Work out the finished part from the listing and answer in its coordinate system (mm). Face numbers are marked on the shaded views. A direction names the side the tool comes from. Coordinates: 2 decimals unless noted, no trailing zeros. Write each loop counter-clockwise with the first axis right and the second up, starting at its lowest first coordinate (ties: lowest second). Pieces come first, ordered by that corner, then holes. Notation, with made-up numbers: (58, -32.5) - (78, -32.5) arc R11 cw to (78, -18.5) - close; hole circle Ø2 at (37.25, 73). An arc over 180 degrees is marked (long way). Use a Markdown table: item, result. Add a question column.
(1) The part is cut by section A-A, the plane z = 6. Give the vertices of the cut face in (x, y) (3 decimals).
(2) Given pin 1 Ø6 at (x, y) = (-3, -27.5) entering from -Z; pin 2 Ø3 at (x, y) = (0, -1) entering from -Z; pin 3 Ø5.5 at (x, z) = (0.5, 9.5) entering from -Y (3 decimals), each flat-ended and moving along its own axis, determine where each tip first touches the part or whether it passes through.
(3) The part is cut by section C-C, the plane x = 0. Give the vertices of the cut face in (y, z) (3 decimals).
(4) Find the intervals of material crossed by line 1 (X direction, y = 0, z = -1); line 2 (X direction, y = -18, z = 12) (3 decimals); line 3 (Z direction, x = 3.75, y = -17) (3 decimals), in increasing order. Write a range as from..to.
(5) The part is cut by section D-D, the plane z = 20.65. Give the vertices of the cut face in (x, y) (3 decimals).
(6) For a pull along Z with two mould halves and no side action, classify the marked faces 4, 5 and 6 as released by +Z, released by -Z, zero draft, split by the parting line, or undercut.
(7) The part is cut by section B-B, the plane y = 0. Give the vertices of the cut face in (x, z) (3 decimals), then the cut area to 3 significant figures.
(8) A tool of negligible diameter and unlimited length cuts with its end or side. For the marked faces 1, 2 and 3, from which of +Z, -Z, +X, -X, +Y, -Y can it reach the whole face along a straight path? Write none if from no direction.
from build123d import *

# Parameters (mm, degrees)
BOSS_EXTRUDE1_DEPTH = 25.4
CUT_EXTRUDE1_DEPTH  = 9.5
SKETCH5_W           = 25.4
SKETCH5_H           = 42.164
BOSS_EXTRUDE2_DEPTH = 11.43
CUT_EXTRUDE2_REACH  = 53.538
CUT_EXTRUDE3_REACH  = 53.255
CUT_EXTRUDE4_DEPTH  = 20
SKETCH10_W          = 19.05
SKETCH10_H          = 19.05
CUT_EXTRUDE5_DEPTH  = 26.289
CUT_EXTRUDE6_REACH  = 55.322
SKETCH11_W          = 1.5875
SKETCH11_H          = 12.7
SKETCH12_R          = 0.9921875
CUT_EXTRUDE7_DEPTH  = 51.724378715
CUT_EXTRUDE8_REACH  = 52.836
SKETCH13_R          = 0.9921875


with BuildPart() as part:
    # Sketch2 → Boss-Extrude1 (new body)
    with BuildSketch(Plane.XY):
        Polygon((12.7, -6.35), (14.2875, -6.35), (14.2875, 6.35), (-14.2875, 6.35), (-14.2875, -6.35), (-12.7, -6.35), (-12.7, -35.814), (12.7, -35.814), align=None)
    extrude(amount=BOSS_EXTRUDE1_DEPTH)

    # Sketch3 → Cut-Extrude1 (cut)
    with BuildSketch(Plane.XY.offset(25.4)):
        with BuildLine():
            Line((2.003122562, 2.3), (2.003122562, -2.3))
            ThreePointArc((2.003122562, -2.3), (-3.05, 0), (2.003122562, 2.3))
        make_face()
    extrude(amount=-CUT_EXTRUDE1_DEPTH, mode=Mode.SUBTRACT)

    # Sketch5 → Boss-Extrude2 (add)
    with BuildSketch(Plane(origin=(0, 0, 0), x_dir=(-1, 0, 0), z_dir=(0, 0, -1))):
        with Locations((0, -14.732)):
            Rectangle(SKETCH5_W, SKETCH5_H)
    extrude(amount=BOSS_EXTRUDE2_DEPTH)

    # Sketch6 → Cut-Extrude2 (cut, up to next)
    with BuildSketch(Plane(origin=(12.7, 0, 0), x_dir=(0, 0, -1), z_dir=(1, 0, 0)), mode=Mode.PRIVATE) as cut_extrude2_sk1:
        Polygon((3.175, -35.814), (11.43, -23.01875), (11.43, -35.814), align=None)
    cut_extrude2_tool1 = extrude(cut_extrude2_sk1.sketch, amount=-CUT_EXTRUDE2_REACH, mode=Mode.PRIVATE) & part.part
    add(cut_extrude2_tool1.solids().sort_by_distance((12.7, -31.548917, -8.678333))[0], mode=Mode.SUBTRACT)

    # Sketch7 → Cut-Extrude3 (cut, up to next)
    with BuildSketch(Plane.XZ.offset(35.814), mode=Mode.PRIVATE) as cut_extrude3_sk1:
        Polygon((-12.7, -11.43), (-12.7, -3.175), (-6.35, -11.43), align=None)
    cut_extrude3_tool1 = extrude(cut_extrude3_sk1.sketch, amount=-CUT_EXTRUDE3_REACH, mode=Mode.PRIVATE) & part.part
    # Sketch7 → Cut-Extrude3 (cut, up to next)
    with BuildSketch(Plane.XZ.offset(35.814), mode=Mode.PRIVATE) as cut_extrude3_sk2:
        Polygon((6.35, -11.43), (12.7, -3.175), (12.7, -11.43), align=None)
    cut_extrude3_tool2 = extrude(cut_extrude3_sk2.sketch, amount=-CUT_EXTRUDE3_REACH, mode=Mode.PRIVATE) & part.part
    add(cut_extrude3_tool1.solids().sort_by_distance((-10.583333, -35.814, -8.678333))[0], mode=Mode.SUBTRACT)
    add(cut_extrude3_tool2.solids().sort_by_distance((10.583333, -35.814, -8.678333))[0], mode=Mode.SUBTRACT)

    # Sketch8 → Cut-Extrude4 (cut)
    with BuildSketch(Plane(origin=(0, 0, -11.43), x_dir=(-1, 0, 0), z_dir=(0, 0, -1))):
        with BuildLine():
            Line((-1.651, 2.859615883), (1.651, 2.859615883))
            ThreePointArc((1.651, 2.859615883), (0, -3.302), (-1.651, 2.859615883))
        make_face()
    extrude(amount=-CUT_EXTRUDE4_DEPTH, mode=Mode.SUBTRACT)

    # Sketch10 → Cut-Extrude5 (cut)
    with BuildSketch(Plane.XZ.offset(35.814)):
        with Locations((0, 12.7)):
            Rectangle(SKETCH10_W, SKETCH10_H)
    extrude(amount=-CUT_EXTRUDE5_DEPTH, mode=Mode.SUBTRACT)

    # Sketch11 → Cut-Extrude6 (cut, up to next)
    with BuildSketch(Plane.XY.offset(25.4), mode=Mode.PRIVATE) as cut_extrude6_sk1:
        with Locations((-13.49375, 0)):
            Rectangle(SKETCH11_W, SKETCH11_H)
    cut_extrude6_tool1 = extrude(cut_extrude6_sk1.sketch, amount=-CUT_EXTRUDE6_REACH, mode=Mode.PRIVATE) & part.part
    # Sketch11 → Cut-Extrude6 (cut, up to next)
    with BuildSketch(Plane.XY.offset(25.4), mode=Mode.PRIVATE) as cut_extrude6_sk2:
        with Locations((13.49375, 0)):
            Rectangle(SKETCH11_W, SKETCH11_H)
    cut_extrude6_tool2 = extrude(cut_extrude6_sk2.sketch, amount=-CUT_EXTRUDE6_REACH, mode=Mode.PRIVATE) & part.part
    add(cut_extrude6_tool1.solids().sort_by_distance((-13.49375, 0, 25.4))[0], mode=Mode.SUBTRACT)
    add(cut_extrude6_tool2.solids().sort_by_distance((13.49375, 0, 25.4))[0], mode=Mode.SUBTRACT)

    # Sketch12 → Cut-Extrude7 (cut, through all)
    with BuildSketch(Plane(origin=(12.7, 0, 0), x_dir=(0, 0, -1), z_dir=(1, 0, 0))):
        with Locations(Location((-20.65, 0, 0), (0, 0, 90))):
            Circle(SKETCH12_R)
    extrude(amount=-CUT_EXTRUDE7_DEPTH, mode=Mode.SUBTRACT)

    # Sketch13 → Cut-Extrude8 (cut, up to next)
    with BuildSketch(Plane(origin=(0, 6.35, 0), x_dir=(1, 0, 0), z_dir=(0, 1, 0)), mode=Mode.PRIVATE) as cut_extrude8_sk1:
        with Locations(Location((0, 1.43, 0), (0, 0, 180))):
            Circle(SKETCH13_R)
    cut_extrude8_tool1 = extrude(cut_extrude8_sk1.sketch, amount=-CUT_EXTRUDE8_REACH, mode=Mode.PRIVATE) & part.part
    add(cut_extrude8_tool1.solids().sort_by_distance((0, 6.35, -1.43))[0], mode=Mode.SUBTRACT)


solid = part.part
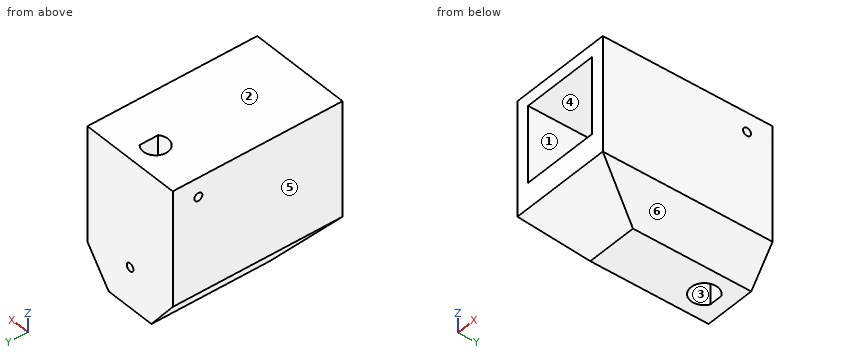
Model answer:
| question | item | result |
|---|---|---|
| 1 | outline | (-12.7, -35.814) - (-9.525, -35.814) - (-9.525, -9.525) - (9.525, -9.525) - (9.525, -35.814) - (12.7, -35.814) - (12.7, 6.35) - (-12.7, 6.35) - close; hole (-1.651, 2.86) arc R3.302 ccw (long way) to (1.651, 2.86) - close |
| 2 | pin 1 | z = -10.47 |
| 2 | pin 2 | z = 8.57 |
| 2 | pin 3 | y = -9.525 |
| 3 | outline | (-35.814, -3.175) - (-23.019, -11.43) - (-3.302, -11.43) - (-3.302, 8.57) - (2.86, 8.57) - (2.86, -0.438) - (6.35, -0.438) - (6.35, 25.4) - (3.05, 25.4) - (3.05, 15.9) - (-3.05, 15.9) - (-3.05, 25.4) - (-35.814, 25.4) - (-35.814, 22.225) - (-9.525, 22.225) - (-9.525, 3.175) - (-35.814, 3.175) - close; (2.86, -11.43) - (6.35, -11.43) - (6.35, -2.422) - (2.86, -2.422) - close |
| 4 | line 1 | -12.7..-3.3, 3.3..12.7 |
| 4 | line 2 | -12.7..-9.525, 9.525..12.7 |
| 4 | line 3 | -11.43..3.175, 22.225..25.4 |
| 5 | outline | (-12.7, -35.814) - (-9.525, -35.814) - (-9.525, -9.525) - (9.525, -9.525) - (9.525, -35.814) - (12.7, -35.814) - (12.7, -0.992) - (2.003, -0.992) - (2.003, -2.3) arc R3.05 cw to (-2.884, -0.992) - (-12.7, -0.992) - close; (-12.7, 0.992) - (-2.884, 0.992) arc R3.05 cw to (2.003, 2.3) - (2.003, 0.992) - (12.7, 0.992) - (12.7, 6.35) - (-12.7, 6.35) - close |
| 6 | face 4 | undercut |
| 6 | face 5 | zero draft |
| 6 | face 6 | released by -Z |
| 7 | outline | (-12.7, -3.175) - (-6.35, -11.43) - (-3.302, -11.43) - (-3.302, 8.57) - (3.302, 8.57) - (3.302, -11.43) - (6.35, -11.43) - (12.7, -3.175) - (12.7, 19.658) - (2.003, 19.658) - (2.003, 15.9) - (-3.05, 15.9) - (-3.05, 19.658) - (-12.7, 19.658) - close; (-12.7, 21.642) - (-3.05, 21.642) - (-3.05, 25.4) - (-12.7, 25.4) - close; (2.003, 21.642) - (12.7, 21.642) - (12.7, 25.4) - (2.003, 25.4) - close |
| 7 | area | 663 mm^2 |
| 8 | face 1 | -Y |
| 8 | face 2 | +Z, +X, -X, +Y, -Y |
| 8 | face 3 | -Z |
